from build123d import *

# Parameters (mm, degrees)
EXTRUDE_1_DEPTH      = 3.75
EXTRUDE_1_DEPTH_BACK = 3.75
SKETCH_2_W           = 3
SKETCH_2_H           = 3
EXTRUDE_2_DEPTH      = 1
EXTRUDE_3_DEPTH      = 2
EXTRUDE_3_DEPTH_BACK = 2
CUT_EXTRUDE_1_REACH  = 16.741
CUT_EXTRUDE_START    = -3
CUT_EXTRUDE_2_DEPTH  = 3
CUT_EXTRUDE_START_2  = -7.5
CUT_EXTRUDE_3_DEPTH  = 3
FILLET_1_R           = 0.2
FILLET_2_R           = 0.1


with BuildPart() as part:
    # 草图1 → 凸台-拉伸1 (new, two sides: drawn at the far end of the back side and taken through both)
    with BuildSketch(Plane.XY.offset(-EXTRUDE_1_DEPTH_BACK)):
        with BuildLine():
            Line((-7.5, 0), (7.5, 0))
            Line((7.5, 0), (3.75, 4))
            Line((3.75, 4), (3.75, 7))
            ThreePointArc((3.75, 7), (2.90473751, 9.371708245), (0.75, 10.674234614))
            Line((0.75, 10.674234614), (0.75, 9.645751311))
            ThreePointArc((0.75, 9.645751311), (0, 4.25), (-0.75, 9.645751311))
            Line((-0.75, 9.645751311), (-0.75, 10.674234614))
            ThreePointArc((-0.75, 10.674234614), (-2.90473751, 9.371708245), (-3.75, 7))
            Line((-3.75, 7), (-3.75, 4))
            Line((-3.75, 4), (-7.5, 0))
        make_face()
    extrude(amount=EXTRUDE_1_DEPTH + EXTRUDE_1_DEPTH_BACK)

    # 草图2 → 凸台-拉伸2 (add)
    with BuildSketch(Plane.XZ):
        Rectangle(SKETCH_2_W, SKETCH_2_H)
    extrude(amount=EXTRUDE_2_DEPTH)

    # 草图3 → 凸台-拉伸3 (add, two sides: drawn at the far end of the back side and taken through both)
    with BuildSketch(Plane.XY.offset(-EXTRUDE_3_DEPTH_BACK)):
        with BuildLine():
            Line((-1.95, -2.5), (1.95, -2.5))
            Line((1.95, -2.5), (1.95, -1.555590279))
            ThreePointArc((1.95, -1.555590279), (1.780042303, -1.088161527), (1.5, -0.677124344))
            Line((1.5, -0.677124344), (-1.5, -0.677124344))
            ThreePointArc((-1.5, -0.677124344), (-1.780042303, -1.088161527), (-1.95, -1.555590279))
            Line((-1.95, -1.555590279), (-1.95, -2.5))
        make_face()
    extrude(amount=EXTRUDE_3_DEPTH + EXTRUDE_3_DEPTH_BACK)

    # 草图4 → 切除-拉伸1 (cut, up to next)
    with BuildSketch(Plane.ZY.offset(1.95), mode=Mode.PRIVATE) as cut_extrude_1_sk1:
        with BuildLine():
            Line((-1.95, -2.5), (-1.95, -1.555590279))
            ThreePointArc((-1.95, -1.555590279), (-1.780042303, -1.088161527), (-1.5, -0.677124344))
            Line((-1.5, -0.677124344), (-2, -0.677124344))
            Line((-2, -0.677124344), (-2, -2.5))
            Line((-2, -2.5), (-1.95, -2.5))
        make_face()
    cut_extrude_1_tool1 = extrude(cut_extrude_1_sk1.sketch, amount=-CUT_EXTRUDE_1_REACH, mode=Mode.PRIVATE) & part.part
    # 草图4 → 切除-拉伸1 (cut, up to next)
    with BuildSketch(Plane.ZY.offset(1.95), mode=Mode.PRIVATE) as cut_extrude_1_sk2:
        with BuildLine():
            Line((1.95, -2.5), (1.95, -1.555590279))
            ThreePointArc((1.95, -1.555590279), (1.780042303, -1.088161527), (1.5, -0.677124344))
            Line((1.5, -0.677124344), (2, -0.677124344))
            Line((2, -0.677124344), (2, -2.5))
            Line((2, -2.5), (1.95, -2.5))
        make_face()
    cut_extrude_1_tool2 = extrude(cut_extrude_1_sk2.sketch, amount=-CUT_EXTRUDE_1_REACH, mode=Mode.PRIVATE) & part.part
    add(cut_extrude_1_tool1.solids().sort_by_distance((-1.95, -1.175075, -1.873038))[0], mode=Mode.SUBTRACT)
    add(cut_extrude_1_tool2.solids().sort_by_distance((-1.95, -1.175075, 1.873038))[0], mode=Mode.SUBTRACT)

    # 草图5 → 切除-拉伸2 (cut)
    with BuildSketch(Plane.XY.offset(3.75).offset(CUT_EXTRUDE_START)):
        with BuildLine():
            Line((-5, 1), (5, 1))
            Line((5, 1), (2.299653235, 4.03789011))
            ThreePointArc((2.299653235, 4.03789011), (0, 3.25), (-2.299653235, 4.03789011))
            Line((-2.299653235, 4.03789011), (-5, 1))
        make_face()
    extrude(amount=CUT_EXTRUDE_2_DEPTH, mode=Mode.SUBTRACT)

    # 草图5<2> → 切除-拉伸3 (cut)
    with BuildSketch(Plane.XY.offset(3.75).offset(CUT_EXTRUDE_START_2)):
        with BuildLine():
            Line((-5, 1), (5, 1))
            Line((5, 1), (2.299653235, 4.03789011))
            ThreePointArc((2.299653235, 4.03789011), (0, 3.25), (-2.299653235, 4.03789011))
            Line((-2.299653235, 4.03789011), (-5, 1))
        make_face()
    extrude(amount=CUT_EXTRUDE_3_DEPTH, mode=Mode.SUBTRACT)

    # 圆角1
    fillet_1_edges = [part.edges().sort_by_distance(p)[0] for p in [
        (7.5, 0, 0),
        (-7.5, 0, 0),
    ]]
    fillet(fillet_1_edges, radius=FILLET_1_R)

    # 圆角2
    fillet_2_edges = [part.edges().sort_by_distance(p)[0] for p in [
        (0, -2.5, 1.95),
        (-1.95, -2.5, 0),
        (1.95, -2.5, 0),
        (0, -2.5, -1.95),
    ]]
    fillet(fillet_2_edges, radius=FILLET_2_R)


solid = part.part
Build history of the part. All positions in model axes, mm. A direction names the side the tool comes from. Round coordinates to 2 decimals unless told otherwise and drop trailing zeros. Order: outer loops, then holes, each group sorted by start corner. A loop starts at its lowest first (then second) coordinate and runs counter-clockwise, first axis right, second up. Notation, with made-up numbers: M 5.5,21 L 17.5,21 A22 ccw 17.5,58 Z; hole C 34.25,47 d2. An arc over 180 degrees is marked long. Use CSV: the item, a comma, the result in double quotes. Start each with the question number.
(1) Tool access for faces 1 (the face through (1.95, -2, 0)), 2 (the face through (-3.75, 6, 0)), 3 (the face through (0, 1, -2)), 4 (the face through (0, -2, 1.95)), 5 (the face through (-1.777, -1.082, -0.027)): list every direction of +Z, -Z, +X, -X, +Y, -Y with a clear straight run to the whole face (end or side of a thin tool).
(2) Cut at B-B on x = 0. List the corners of the cut face in (y, z).
(3) Cut at C-C on z = 3. List the corners of the cut face in (x, y), then the cut area to 3 significant figures.
(4) Drill centre lines: probe 1 along X at (y, z) = (7, 1.5); probe 2 along Y at (x, z) = (0, 1.25); probe 3 along Y at (x, z) = (0, -2). Where is each one in solid material? Low to high.
(5) Flat gauge pins, fed straight in: P1, Ø0.5, axis at y = -0.5, z = 0, coming from the -X side; P2, Ø1.5, axis at y = 5, z = 0, coming from the +X side; P3, Ø3.5, axis at y = 5.5, z = 0.5, coming from the -X side. Where does each tip first touch, or does it go through?
(6) Cut at A-A on y = 8.5. List the corners of the cut face in (x, z).
(7) Mould opens along X. For faces 6 (the face through (0.11, 4.252, -0.053)), 7 (the face through (1.78, -1.09, -0.03)), 8 (the face through (0, 4, -3.75)) say: +X half, -X half, draft (parallel to the pull), parting line (faces both ways), or undercut.
(8) Cut at D-D on z = -0.25. List the corners of the cut face in (x, y), then the cut area to 3 significant figures.
Findings:
1,face 1,"+Z, -Z, +X, -Y"
1,face 2,"+Z, -Z, -X, +Y"
1,face 3,"-Z"
1,face 4,"+Z, +X, -X, -Y"
1,face 5,"+Z, -Z, -X"
2,outline,"M -2.5,-1.85 A0.1 ccw -2.4,-1.95 L -1.56,-1.95 A2 ccw -0.68,-1.5 L 0,-1.5 L 0,-3.75 L 1,-3.75 L 1,-0.75 L 3.25,-0.75 L 3.25,-3.75 L 4.25,-3.75 L 4.25,3.75 L 3.25,3.75 L 3.25,0.75 L 1,0.75 L 1,3.75 L 0,3.75 L 0,1.5 L -0.68,1.5 A2 ccw -1.56,1.95 L -2.4,1.95 A0.1 ccw -2.5,1.85 Z"
3,outline,"M -7.18,0.34 A0.2 ccw -7.04,0 L 7.04,0 A0.2 ccw 7.18,0.34 L 3.75,4 L 3.75,7 A3.75 ccw 0.75,10.67 L 0.75,9.65 A2.75 cw long -0.75,9.65 L -0.75,10.67 A3.75 ccw -3.75,7 L -3.75,4 Z; hole M -5,1 L 5,1 L 2.3,4.04 A3.75 cw -2.3,4.04 Z"
3,area,"44.5 mm^2"
4,probe 1,"x = -3.75 to -2.75, 2.75 to 3.75"
4,probe 2,"y = -2.5 to 1, 3.25 to 4.25"
4,probe 3,"y = 0 to 1, 3.25 to 4.25"
5,P1,"stops at x = -1.56"
5,P2,"stops at x = 3.75"
5,P3,"stops at x = -3.98"
6,outline,"M -3.44,-3.75 L -2.3,-3.75 L -2.3,3.75 L -3.44,3.75 Z; M 2.3,-3.75 L 3.44,-3.75 L 3.44,3.75 L 2.3,3.75 Z"
7,face 6,"undercut"
7,face 7,"+X half"
7,face 8,"draft"
8,outline,"M -7.18,0.34 A0.2 ccw -7.04,0 L -1.5,0 L -1.5,-0.68 A2 ccw -1.95,-1.56 L -1.95,-2.4 A0.1 ccw -1.85,-2.5 L 1.85,-2.5 A0.1 ccw 1.95,-2.4 L 1.95,-1.56 A2 ccw 1.5,-0.68 L 1.5,0 L 7.04,0 A0.2 ccw 7.18,0.34 L 3.75,4 L 3.75,7 A3.75 ccw 0.75,10.67 L 0.75,9.65 A2.75 cw long -0.75,9.65 L -0.75,10.67 A3.75 ccw -3.75,7 L -3.75,4 Z"
8,area,"73.0 mm^2"
